```python
from build123d import *

# Parameters (mm, degrees)
F1_DEPTH = 80
F2_T     = -2.5
F3_SIZE  = 2


with BuildPart() as f1:
    # F0 (on Front) → F1 (new body)
    with BuildSketch(Plane.XZ):
        with BuildLine():
            Line((30, 100), (-30, 100))
            ThreePointArc((-30, 100), (-44.142136, 94.142136), (-50, 80))
            Line((-50, 80), (-50, -100))
            Line((-50, -100), (50, -100))
            Line((50, -100), (50, 80))
            ThreePointArc((50, 80), (44.142136, 94.142136), (30, 100))
        make_face()
    extrude(amount=F1_DEPTH)

    # F2
    f2_openings = [f1.faces().sort_by_distance(p)[0] for p in [
        (0, -80, -0.82716),
    ]]
    offset(amount=F2_T, openings=f2_openings)

    # F3
    f3_edges = [f1.edges().sort_by_distance(p)[0] for p in [
        (50, 0, -10),
        (0, 0, 100),
        (-44.142136, 0, 94.142136),
        (-50, 0, -10),
        (0, 0, -100),
        (44.142136, 0, 94.142136),
    ]]
    chamfer(f3_edges, length=F3_SIZE)


solid = f1.part
```
Verification items for the finished model (mm, model axes). A direction names the side the tool comes from. Round coordinates to 2 decimals unless told otherwise and drop trailing zeros. Write each loop counter-clockwise with the first axis right and the second up, starting at its lowest first coordinate (ties: lowest second). Pieces come first, ordered by that corner, then holes. Notation, with made-up numbers: (28, -36) - (33, -36) arc R27 cw to (33, -8) - close; hole circle Ø4 at (65.25, 68). An arc over 180 degrees is marked (long way). Answer as a JSON object with one key per item and string values. Group by question number.
Q1. Go/stop test with flat-tipped pins: pin 1 Ø12 at (x, y) = (37.5, -27) entering from +Z; pin 2 Ø8 at (x, z) = (-18, 56) entering from -Y. Record where each tip stops, or that it passes through.
Q2. Section check A-A, the plane y = -42.5. Enter the section's corners in (x, z).
Q3. Section check C-C, the plane x = -6. Enter the section's corners in (y, z), plus the area to 4 significant figures.
Q4. Mould release check, pull along X, two halves, no side actions. Record for faces 3 (the flat face through (47.5, -41, -10)), 4 (the cylindrical face through (44.297, -40.454, 93.986)), 5 (the flat face through (-1, -41, -97.5)), 6 (the conical face through (-42.81, -0.32, 93.1)): released by +X, released by -X, zero draft, split by the parting line, or undercut.
Q5. Thickness scan on line 1 (Z direction, x = -17, y = -70); line 2 (X direction, y = -4, z = -37.5); line 3 (Y direction, x = -3.5, z = 56). Record the ranges inside material, lowest first.
Q6. Tool access check on faces 1 (the flat face through (50, -40, -11)), 2 (the flat face through (-47.5, -41, -8)). Record the directions out of +Z, -Z, +X, -X, +Y, -Y that give a thin tool (end or side, any length) a straight path to the whole face; none if there is none.
Q7. Section check B-B, the plane z = -48.5. Enter the section's corners in (x, y), plus the area to 4 significant figures.
Found:
{
 "1": {"pin 1": "stops at z = 99.94", "pin 2": "stops at y = -2.5"},
 "2": {"outline": "(-50, -100) - (50, -100) - (50, 80) arc R20 ccw to (30, 100) - (-30, 100) arc R20 ccw to (-50, 80) - close; hole (-47.5, -97.5) - (47.5, -97.5) - (47.5, 80) arc R17.5 ccw to (30, 97.5) - (-30, 97.5) arc R17.5 ccw to (-47.5, 80) - close"},
 "3": {"outline": "(-80, -100) - (-2, -100) - (0, -98) - (0, 98) - (-2, 100) - (-80, 100) - (-80, 97.5) - (-2.5, 97.5) - (-2.5, -97.5) - (-80, -97.5) - close", "area": "883.5 mm^2"},
 "4": {"face 3": "undercut", "face 4": "released by +X", "face 5": "undercut", "face 6": "released by -X"},
 "5": {"line 1": "z = -100 to -97.5, 97.5 to 100", "line 2": "x = -50 to -47.5, 47.5 to 50", "line 3": "y = -2.5 to 0"},
 "6": {"face 1": "+Z, -Z, +X, +Y, -Y", "face 2": "-Y"},
 "7": {"outline": "(-50, -80) - (-47.5, -80) - (-47.5, -2.5) - (47.5, -2.5) - (47.5, -80) - (50, -80) - (50, -2) - (48, 0) - (-48, 0) - (-50, -2) - close", "area": "633.5 mm^2"}
}
